```python
from build123d import *

# Parameters (mm, degrees)
SKETCH_1_W          = 160
SKETCH_1_H          = 111
SKETCH_1_R          = 2
SKETCH_1_R_2        = 1.5
EXTRUDE_1_DEPTH     = 4
SKETCH_2_W          = 160
SKETCH_2_H          = 111
SKETCH_2_W_2        = 154
SKETCH_2_H_2        = 105
EXTRUDE_4_DEPTH     = 50
SKETCH_3_R          = 2.5
SKETCH_3_R_2        = 1.5
EXTRUDE_5_DEPTH     = 15
SKETCH_4_R          = 5
CUT_EXTRUDE_1_DEPTH = 5


with BuildPart() as part:
    # Sketch 1 → Extrude 1 (new body)
    with BuildSketch(Plane(origin=(0, 0, 0), x_dir=(1, 0, 0), z_dir=(0, 1, 0))):
        with Locations((-1.924564797, 0)):
            Rectangle(SKETCH_1_W, SKETCH_1_H)
        with Locations(Location((-71.924564797, 44.9, 0), (0, 0, 270))):
            Circle(SKETCH_1_R, mode=Mode.SUBTRACT)
        with Locations(Location((-71.924564797, -44.9, 0), (0, 0, 90))):
            Circle(SKETCH_1_R, mode=Mode.SUBTRACT)
        with Locations(Location((-2.124564797, 44.9, 0), (0, 0, 270))):
            Circle(SKETCH_1_R, mode=Mode.SUBTRACT)
        with Locations(Location((-2.124564797, -44.9, 0), (0, 0, 90))):
            Circle(SKETCH_1_R, mode=Mode.SUBTRACT)
        with Locations(Location((-26.124564797, 48.16, 0), (0, 0, 270))):
            Circle(SKETCH_1_R_2, mode=Mode.SUBTRACT)
        with Locations(Location((-26.124564797, 27.96, 0), (0, 0, 270))):
            Circle(SKETCH_1_R_2, mode=Mode.SUBTRACT)
    extrude(amount=EXTRUDE_1_DEPTH)



with BuildPart() as body_2:
    # Sketch 2 → Extrude 4 (new body)
    with BuildSketch(Plane(origin=(0, 4, 0), x_dir=(1, 0, 0), z_dir=(0, 1, 0))):
        with Locations((-1.924564797, 0)):
            Rectangle(SKETCH_2_W, SKETCH_2_H)
        with Locations((-1.924564797, 0)):
            Rectangle(SKETCH_2_W_2, SKETCH_2_H_2, mode=Mode.SUBTRACT)
    extrude(amount=EXTRUDE_4_DEPTH)


with BuildPart() as part_1:
    add(part.part)

    add(body_2.part)  # Extrude 5 merges body 2
    # Sketch 3 → Extrude 5 (add)
    # profile 1 of 2: a face of its own
    with BuildSketch(Plane(origin=(0, 4, 0), x_dir=(1, 0, 0), z_dir=(0, 1, 0))):
        with Locations(Location((-26.124564797, 48.16, 0), (0, 0, 270))):
            Circle(SKETCH_3_R)
        with Locations(Location((-26.124564797, 48.16, 0), (0, 0, 270))):
            Circle(SKETCH_3_R_2, mode=Mode.SUBTRACT)
    # profile 2 of 2: a face of its own
    with BuildSketch(Plane(origin=(0, 4, 0), x_dir=(1, 0, 0), z_dir=(0, 1, 0))):
        with Locations(Location((-26.124564797, 27.96, 0), (0, 0, 270))):
            Circle(SKETCH_3_R)
        with Locations(Location((-26.124564797, 27.96, 0), (0, 0, 270))):
            Circle(SKETCH_3_R_2, mode=Mode.SUBTRACT)
    extrude(amount=EXTRUDE_5_DEPTH)

    # Sketch 4 → Cut-Extrude 1 (cut)
    with BuildSketch(Plane.ZY.offset(81.924564797)):
        with Locations((-31, 12.58)):
            Circle(SKETCH_4_R)
    extrude(amount=-CUT_EXTRUDE_1_DEPTH, mode=Mode.SUBTRACT)


solid = part_1.part
```
Here's how the part is built. I have some questions about the finished solid (model axes, mm). A direction names the side the tool comes from. Coordinates: 2 decimals unless noted, no trailing zeros. Order: outer loops, then holes, each group sorted by start corner. A loop starts at its lowest first (then second) coordinate and runs counter-clockwise, first axis right, second up.
Item 1: I'm going to push flat-ended pins straight in: pin 1 Ø6.5 at (x, z) = (-71.92, 44.9) entering from +Y; pin 2 Ø1.5 at (x, z) = (-27.5, -28.5) entering from +Y; pin 3 Ø9 at (y, z) = (12.58, -31) entering from -X. Where does each tip first touch, or does it pass through?
Response values:
pin 1: stops at y = 4
pin 2: stops at y = 19
pin 3: stops at x = -28.62
Item 2: If we section it at A-A, the plane y = 12.58: List the corners of the cut face in (x, z) for me, then the cut area to 3 significant figures.
Response values:
outline: (-81.92, -55.5) - (78.08, -55.5) - (78.08, 55.5) - (-81.92, 55.5) - (-81.92, -26) - (-78.92, -26) - (-78.92, 52.5) - (75.08, 52.5) - (75.08, -52.5) - (-78.92, -52.5) - (-78.92, -36) - (-81.92, -36) - close; circle Ø5 at (-26.12, -48.16); circle Ø5 at (-26.12, -27.96); hole circle Ø3 at (-26.12, -48.16); hole circle Ø3 at (-26.12, -27.96)
area: 1,590 mm2
Item 3: If we section it at C-C, the plane y = 42.5: List the corners of the cut face in (x, z) for me.
Response values:
outline: (-81.92, -55.5) - (78.08, -55.5) - (78.08, 55.5) - (-81.92, 55.5) - close; hole (-78.92, -52.5) - (75.08, -52.5) - (75.08, 52.5) - (-78.92, 52.5) - close
Item 4: I need wall thicknesses on probe 1 along Z at (x, y) = (49, 37.5); probe 2 along X at (y, z) = (47, 8); probe 3 along Y at (x, z) = (-16.5, 17.5). Which ranges of each line are inside material? Lowest first, please.
Response values:
probe 1: z = -55.5 to -52.5, 52.5 to 55.5
probe 2: x = -81.92 to -78.92, 75.08 to 78.08
probe 3: y = 0 to 4
Item 5: If we section it at D-D, the plane x = 41.5: List the corners of the cut face in (y, z) for me.
Response values:
outline: (0, -55.5) - (54, -55.5) - (54, -52.5) - (4, -52.5) - (4, 52.5) - (54, 52.5) - (54, 55.5) - (0, 55.5) - close
Item 6: Thinking about a two-plate mould opening in Y: for faces 3 (the face through (-28, 19, -48)), 4 (the face through (-2.04, 1.97, -46.9)), 5 (the face through (-80.446, 15.959, -34.685)), which applies, pulls with the +Y half, pulls with the -Y half, needs draft (parallel to the pull), parting line crosses it, or undercut?
Response values:
face 3: pulls with the +Y half
face 4: needs draft
face 5: undercut
Item 7: If we section it at B-B, the plane z = 44.9: List the corners of the cut face in (x, y) for me.
Response values:
outline: (-81.92, 0) - (-73.92, 0) - (-73.92, 4) - (-78.92, 4) - (-78.92, 54) - (-81.92, 54) - close; (-69.92, 0) - (-4.12, 0) - (-4.12, 4) - (-69.92, 4) - close; (-0.12, 0) - (78.08, 0) - (78.08, 54) - (75.08, 54) - (75.08, 4) - (-0.12, 4) - close
Item 8: Which directions (+Z, -Z, +X, -X, +Y, -Y) give clear straight access to the entire face, cutting with the end or side of a thin tool? Please do faces 1 (the face through (-69.94, 1.97, -45.16)), 2 (the face through (-27.08, 11.4, -45.85)).
Response values:
face 1: +Y, -Y
face 2: +Y
